Autodesk Inventor part; units mm, degrees
ref_plane "YZ Plane" through (0, 0, 0) normal (1, 0, 0) x (0, 1, 0)
ref_plane "XY Plane" through (0, 0, 0) normal (0, 0, 1) x (1, 0, 0)
ref_plane "MountingScrew" through (0, 0, 0) normal (0, 1, 0) x (-1, 0, 0)
ref_plane "Bracketheight" through (0, 15, 0) normal (0, 1, 0) x (-1, 0, 0)
sketch "Sketch1" plane through (0, 0, 0) normal (0, 0, 1) x (1, 0, 0)
  line L0 (0, -15.05) -> (20, -15.05)
  line L1 (20, -15.05) -> (20, 15)
  line L2 (20, 15) -> (0, 15)
  line L3 (0, 15) -> (0, -15.05)
  circle A0 centre (6, 0) radius 2.75 construction
  line L4 (0, -2.75) -> (20, -2.75) construction
  line L5 (3.25, 15) -> (3.25, -15.05) construction
  line L6 (-4, 0) -> (24, 0) construction
  line L7 (0, 21.01) -> (0, -21.06) construction
  line L8 (-4, 15) -> (24, 15) construction
  dimension "d0" = 5.5
  dimension "d1" = 12.3
  dimension "d2" = 3.25
  dimension "d31" = 6
  dimension "d36" = 20
extrude "Extrusion1" add sketch "Sketch1" along normal blind 4
sketch "Sketch2" plane through (0, 0, 4) normal (0, 0, 1) x (1, 0, 0)
  point P0 (0, 0)
  point P1 (6, 0)
hole "Hole1" at (6, 0, 4) direction (0, 0, -1) diameter 5.3 end through all
sketch "Sketch5" plane through (0, 15, 0) normal (0, 1, 0) x (1, 0, 0)
  line L0 (0, 12) -> (20, 12)
  line L1 (20, 12) -> (20, -20)
  line L2 (20, -20) -> (0, -20)
  line L3 (0, -20) -> (0, 12)
  line L4 (20, 0) -> (0, 0) construction
  line L5 (20, 0) -> (0, 0) construction
  line L6 (0, 0) -> (0, -4) construction
  line L7 (20, 0) -> (20, -4) construction
  dimension "d2" = 3.25
  dimension "d60" = 20
  dimension "d61" = 12
extrude "Extrusion4" add sketch "Sketch5" along normal blind 1
sketch "Sketch6" plane through (0, -15.05, 0) normal (-1, 0, 0) x (0, 0, 1)
  line L0 (-12, 30.05) -> (0, 30.05)
  line L1 (-12, 30.05) -> (20, 30.05)
  line L2 (20, 30.05) -> (20, 40.05)
  line L3 (20, 40.05) -> (-12, 40.05)
  line L4 (-12, 40.05) -> (-12, 30.05)
  line L5 (20, 30.05) -> (20, 31.05) construction
  point P0 (0, 15.05)
  dimension "d37" = 10
extrude "Extrusion5" add sketch "Sketch6" against normal blind 2
sketch "Sketch8" plane through (5.5, 0, 4) normal (0, 0, 1) x (1, 0, 0)
  line L0 (-1.8671, 4.1) -> (2.8671, 4.1)
  line L1 (2.8671, 4.1) -> (5.2343, 0)
  line L2 (5.2343, 0) -> (2.8671, -4.1)
  line L3 (2.8671, -4.1) -> (-1.8671, -4.1)
  line L4 (-1.8671, -4.1) -> (-4.2343, 0)
  line L5 (-4.2343, 0) -> (-1.8671, 4.1)
  point P0 (-5.5, 0)
  point P1 (0.5, 0)
  point P2 (0.5, 0)
  dimension "d42" = 8.2
extrude "Extrusion7" cut sketch "Sketch8" against normal blind 2
sketch "Sketch10" plane through (0, -15.05, 0) normal (-1, 0, 0) x (0, 0, 1)
  line L0 (-7.7, 36.75) -> (15.7, 36.75) construction
  line L1 (-7.7, 35.45) -> (15.7, 35.45)
  line L2 (15.7, 38.05) -> (-7.7, 38.05)
  arc A0 (-7.7, 38.05) -> (-7.7, 35.45) centre (-7.7, 36.75) ccw
  arc A1 (15.7, 35.45) -> (15.7, 38.05) centre (15.7, 36.75) ccw
  line L3 (-12, 30.05) -> (-12, 40.05)
  line L4 (0, 30.05) -> (0, 0)
  line L5 (0, 30.05) -> (0, 0)
  line L6 (20, 40.05) -> (-12, 40.05)
  line L7 (20, 30.05) -> (20, 40.05)
  point P0 (0, 15.05)
  point P1 (4, 36.75)
  point P2 (-12, 35.05)
  dimension "d55" = 2.6
  dimension "d59" = 2
  dimension "d63" = 4.3
  dimension "d64" = 4.3
extrude "Extrusion9" cut sketch "Sketch10" against normal through all
sketch "Sketch7" plane through (0, 15, 0) normal (0, -1, 0) x (1, 0, 0)
  line L0 (20, 4) -> (0, 4)
  line L1 (0, 4) -> (0, 20)
  line L2 (20, 4) -> (0, 4)
  line L3 (0, 4) -> (0, 20)
  line L4 (0, 20) -> (20, 20)
  line L5 (20, 20) -> (20, 4)
  point P0 (0, 0)
  dimension "d45" = 5.1
  dimension "d16" = 2.5
  dimension "d17" = 4.25
  dimension "d18" = 8
sketch "Sketch4" plane through (25.5, -5.5, 0) normal (1, 0, 0) x (0, 0, -1)
  line L0 (-5.45, 24.0278) -> (-8, 22.5555)
  line L1 (-8, 22.5555) -> (-10.55, 24.0278)
  line L2 (-10.55, 24.0278) -> (-10.55, 26.9722)
  line L3 (-10.55, 26.9722) -> (-8, 28.4445)
  line L4 (-8, 28.4445) -> (-5.45, 26.9722)
  line L5 (-5.45, 26.9722) -> (-5.45, 24.0278)
  point P0 (0, 5.5)
  point P1 (-8, 25.5)
  point P2 (-8, 25.5)
  dimension "d28" = 5.1
equation "\"d36\" = Schraubenlaenge"
equation "\"d64\" = d63"
equation "\"Schraubenlaenge\" = 20"
properties part number "Enoder_Mount1"
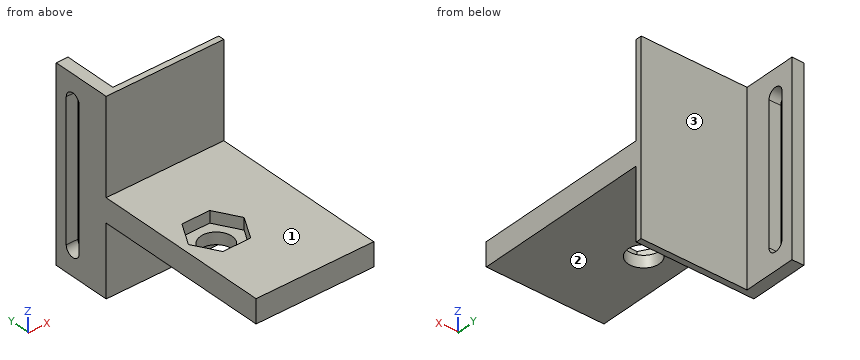
The model under review builds one solid part; all positions refer to its coordinate system, in mm. Face numbers are marked on the shaded views. A direction names the side the tool comes from. Coordinates: 2 decimals unless noted, no trailing zeros. Write each loop counter-clockwise with the first axis right and the second up, starting at its lowest first coordinate (ties: lowest second). Pieces come first, ordered by that corner, then holes. Notation, with made-up numbers: (-27, 47.25) - (-17, 47.25) arc R16 ccw to (-17, 56.25) - close; hole circle Ø5 at (24, -24). An arc over 180 degrees is marked (long way). Answer in a Markdown table with one row per item. Add a question column.
Q1. To check wall thickness, follow line 1 along Y through (x, z) = (6, 1.35); line 2 along X through (y, z) = (0, 1); line 3 along Z through (x, y) = (3, 3.5). State the ranges of each line that lie inside material, in increasing order. Write a range as from..to.
Q2. Consider section B-B on x = 6. Give the boundary of the cut face in (y, z).
Q3. Consider section A-A on y = 21.7. Give the boundary of the cut face in (x, z).
Q4. Clearance check with flat-ended pins moving along their axes: pin 1 (5 mm diameter, centred on x = 15.5, y = 17, fed in from +Z); pin 2 (2 mm diameter, centred on y = 12.5, z = 12, fed in from +X); pin 3 (2.5 mm diameter, centred on y = 22.5, z = 0.5, fed in from +X); pin 4 (2 mm diameter, centred on x = 14, y = -8.5, fed in from +Z). State where each tip first meets the part, or that it passes through.
Q5. For the marked faces 1, 2 and 3, list the 3-axis set-ups (+Z, -Z, +X, -X, +Y, -Y) from which the entire face can be reached by the end or side of a thin tool; tool diameter is ignored.
Q6. Consider section D-D on x = 12. Give the boundary of the cut face in (y, z), then the cut area to 3 significant figures.
Q7. Consider section C-C on z = -5.5. Give the boundary of the cut face in (x, y).
Answers below:
| question | item | result |
|---|---|---|
| 1 | line 1 | -15.05..-2.65, 2.65..16 |
| 1 | line 2 | 0..3.35, 8.65..20 |
| 1 | line 3 | 0..4 |
| 2 | outline | (-15.05, 0) - (-2.65, 0) - (-2.65, 2) - (-4.1, 2) - (-4.1, 4) - (-15.05, 4) - close; (2.65, 0) - (15, 0) - (15, -12) - (16, -12) - (16, 20) - (15, 20) - (15, 4) - (4.1, 4) - (4.1, 2) - (2.65, 2) - close |
| 3 | outline | (0, -12) - (2, -12) - (2, -9) - (0, -9) - close; (0, 17) - (2, 17) - (2, 20) - (0, 20) - close |
| 4 | pin 1 | z = 20 |
| 4 | pin 2 | through |
| 4 | pin 3 | x = 2 |
| 4 | pin 4 | z = 4 |
| 5 | face 1 | +Z, +X, -X, -Y |
| 5 | face 2 | -Z, +X, -X, -Y |
| 5 | face 3 | +Z, -Z, +X, +Y |
| 6 | outline | (-15.05, 0) - (15, 0) - (15, -12) - (16, -12) - (16, 20) - (15, 20) - (15, 4) - (-15.05, 4) - close |
| 6 | area | 152 mm² |
| 7 | outline | (0, 15) - (20, 15) - (20, 16) - (2, 16) - (2, 20.4) - (0, 20.4) - close; (0, 23) - (2, 23) - (2, 25) - (0, 25) - close |
